For this review, take the finished solid that the model builds, in its own axes (mm). Face numbers are marked on the shaded views. A direction names the side the tool comes from. Round coordinates to 2 decimals unless told otherwise and drop trailing zeros. Order: outer loops, then holes, each group sorted by start corner. A loop starts at its lowest first (then second) coordinate and runs counter-clockwise, first axis right, second up. Notation, with made-up numbers: (2.25, 80) -> (52.25, 80) arc R18 cw to (52.25, 97) -> close; hole circle Ø4 at (16.25, 64.5). An arc over 180 degrees is marked (long way). Answer in a Markdown table with one row per item.
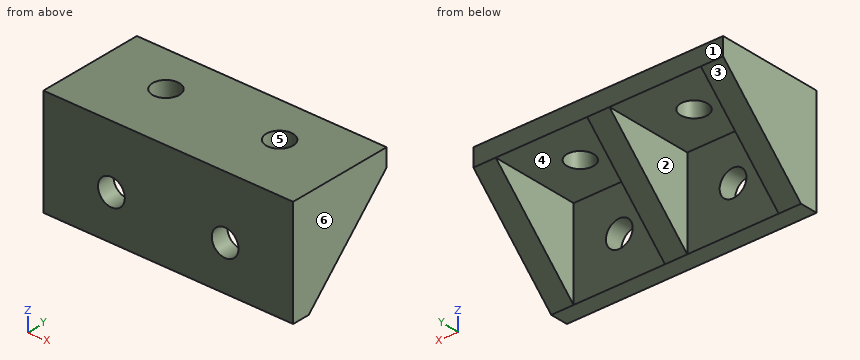
```python
from build123d import *

# Parameters (mm, degrees)
CROQUIS1_R                   = 2.5
SALIENTE_EXTRUIR1_DEPTH      = 4
CROQUIS2_W                   = 50
CROQUIS2_H                   = 4
SALIENTE_EXTRUIR2_DEPTH      = 20
SALIENTE_EXTRUIR3_DEPTH      = 3
SALIENTE_EXTRUIR3_DEPTH_BACK = 53
CROQUIS4_W                   = 20.5
CROQUIS4_H                   = 20
CORTAR_EXTRUIR1_DEPTH        = 20
CROQUIS5_R                   = 3
CORTAR_EXTRUIR2_DEPTH        = 17
CROQUIS6_R                   = 3
CORTAR_EXTRUIR3_DEPTH        = 20


with BuildPart() as part:
    # Croquis1 → Saliente-Extruir1 (new body)
    with BuildSketch(Plane(origin=(0, 0, 0), x_dir=(1, 0, 0), z_dir=(0, 1, 0))):
        Polygon((0, 0), (0, 20), (50, 20), (50, 0), (50, -4), (0, -4), align=None)
        with Locations(Location((12.5, 10, 0), (0, 0, 270))):
            Circle(CROQUIS1_R, mode=Mode.SUBTRACT)
        with Locations(Location((37.5, 10, 0), (0, 0, 270))):
            Circle(CROQUIS1_R, mode=Mode.SUBTRACT)
    extrude(amount=SALIENTE_EXTRUIR1_DEPTH)

    # Croquis2 → Saliente-Extruir2 (add)
    with BuildSketch(Plane(origin=(0, 4, 0), x_dir=(1, 0, 0), z_dir=(0, 1, 0))):
        with Locations((25, -2)):
            Rectangle(CROQUIS2_W, CROQUIS2_H)
    extrude(amount=SALIENTE_EXTRUIR2_DEPTH)

    # Croquis3 → Saliente-Extruir3 (add, two sides: drawn at the far end of the back side and taken through both)
    with BuildSketch(Plane.ZY.offset(-SALIENTE_EXTRUIR3_DEPTH_BACK)):
        Polygon((-20, 4), (-20, 0), (4, 0), (4, 24), (0, 24), align=None)
    extrude(amount=SALIENTE_EXTRUIR3_DEPTH + SALIENTE_EXTRUIR3_DEPTH_BACK)

    # Croquis4 → Cortar-Extruir1 (cut)
    with BuildSketch(Plane(origin=(0, 0, -20), x_dir=(-1, 0, 0), z_dir=(0, 0, -1))):
        with Locations((-37.75, 14)):
            Rectangle(CROQUIS4_W, CROQUIS4_H)
        with Locations((-12.25, 14)):
            Rectangle(CROQUIS4_W, CROQUIS4_H)
    extrude(amount=-CORTAR_EXTRUIR1_DEPTH, mode=Mode.SUBTRACT)

    # Croquis5 → Cortar-Extruir2 (cut)
    with BuildSketch(Plane(origin=(0, 0, 0), x_dir=(-1, 0, 0), z_dir=(0, 0, -1))):
        with Locations((-37.75, 14)):
            Circle(CROQUIS5_R)
        with Locations((-12.25, 14)):
            Circle(CROQUIS5_R)
    extrude(amount=-CORTAR_EXTRUIR2_DEPTH, mode=Mode.SUBTRACT)

    # Croquis6 → Cortar-Extruir3 (cut)
    with BuildSketch(Plane(origin=(0, 4, 0), x_dir=(1, 0, 0), z_dir=(0, 1, 0))):
        with Locations(Location((12.25, 10, 0), (0, 0, 180))):
            Circle(CROQUIS6_R)
        with Locations(Location((37.75, 10, 0), (0, 0, 270))):
            Circle(CROQUIS6_R)
    extrude(amount=-CORTAR_EXTRUIR3_DEPTH, mode=Mode.SUBTRACT)


solid = part.part
```
Q1. Take a section at D-D, the plane y = 15. Write out the cut boundary in (x, z), then the cut area to 3 significant figures.
Answer key:
| item | result |
|---|---|
| outline | (-3, -9) -> (2, -9) -> (2, 0) -> (9.42, 0) -> (9.42, 4) -> (-3, 4) -> close; (15.08, 0) -> (22.5, 0) -> (22.5, -9) -> (27.5, -9) -> (27.5, 0) -> (34.92, 0) -> (34.92, 4) -> (15.08, 4) -> close; (40.58, 0) -> (48, 0) -> (48, -9) -> (53, -9) -> (53, 4) -> (40.58, 4) -> close |
| area | 314 mm^2 |
Q2. Take a section at B-B, the plane x = 12.25. Write out the cut boundary in (y, z).
Answer key:
| item | result |
|---|---|
| outline | (0, -20) -> (4, -20) -> (4, -13) -> (0, -13) -> close; (0, -7) -> (4, -7) -> (4, 0) -> (11, 0) -> (11, 4) -> (0, 4) -> close; (17, 0) -> (24, 0) -> (24, 4) -> (17, 4) -> close |
Q3. To check wall thickness, follow probe 1 along X at (y, z) = (15.75, -6); probe 2 along Z at (x, y) = (12.25, 1.5); probe 3 along Y at (x, z) = (12.25, 1.2). State the ranges of each line that lie inside material, in increasing order.
Answer key:
| item | result |
|---|---|
| probe 1 | x = -3 to 2, 22.5 to 27.5, 48 to 53 |
| probe 2 | z = -20 to -13, -7 to 4 |
| probe 3 | y = 0 to 11, 17 to 24 |
Q4. Tool access review of the marked faces 1 and 2: name each direction out of +Z, -Z, +X, -X, +Y, -Y from which nothing blocks a thin tool from reaching the whole face with its end or side.
Answer key:
| item | result |
|---|---|
| face 1 | +Z, -Z, +X, -X, +Y |
| face 2 | -Z, +Y |
Q5. Clearance check with flat-ended pins moving along their axes: pin 1 Ø1.5 at (x, y) = (39.5, 14.5) entering from +Z; pin 2 Ø9.5 at (x, y) = (37.75, 14) entering from -Z; pin 3 Ø7 at (x, z) = (37.75, -10) entering from +Y. State where each tip first meets the part, or that it passes through.
Answer key:
| item | result |
|---|---|
| pin 1 | passes through |
| pin 2 | stops at z = 0 |
| pin 3 | stops at y = 4 |
Q6. Take a section at A-A, the plane z = -10. Write out the cut boundary in (x, y).
Answer key:
| item | result |
|---|---|
| outline | (-3, 0) -> (9.25, 0) -> (9.25, 4) -> (2, 4) -> (2, 14) -> (-3, 14) -> close; (15.25, 0) -> (34.75, 0) -> (34.75, 4) -> (27.5, 4) -> (27.5, 14) -> (22.5, 14) -> (22.5, 4) -> (15.25, 4) -> close; (40.75, 0) -> (53, 0) -> (53, 14) -> (48, 14) -> (48, 4) -> (40.75, 4) -> close |
Q7. The part is to be moulded in two halves that separate along X. For the marked faces 3, 4, 5 and 6, say which applies: +X half, -X half, draft (parallel to the pull), parting line (faces both ways), or undercut.
Answer key:
| item | result |
|---|---|
| face 3 | draft |
| face 4 | undercut |
| face 5 | undercut |
| face 6 | +X half |
Q8. Take a section at C-C, the plane y = 18.5. Write out the cut boundary in (x, z), then the cut area to 4 significant figures.
Answer key:
| item | result |
|---|---|
| outline | (-3, -5.5) -> (2, -5.5) -> (2, 0) -> (22.5, 0) -> (22.5, -5.5) -> (27.5, -5.5) -> (27.5, 0) -> (48, 0) -> (48, -5.5) -> (53, -5.5) -> (53, 4) -> (-3, 4) -> close |
| area | 306.5 mm^2 |
